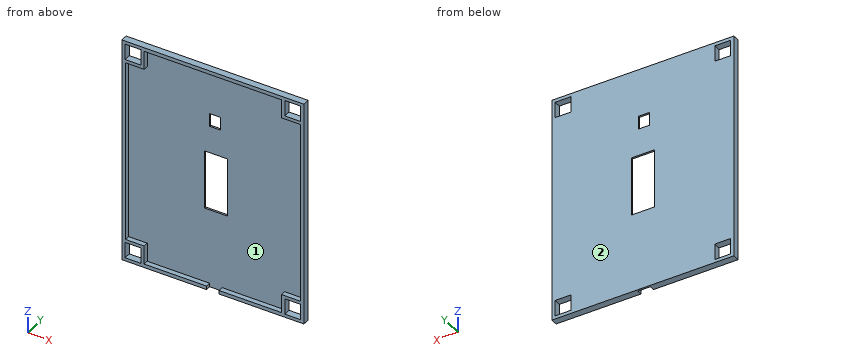
from build123d import *

# Parameters (mm, degrees)
SKETCH1_W           = 80
SKETCH1_H           = 100
BOSS_EXTRUDE1_DEPTH = 3
SKETCH2_W           = 76.8
SKETCH2_H           = 96.8
CUT_EXTRUDE1_DEPTH  = 2.2
CUT_EXTRUDE2_REACH  = 5
SKETCH5_W           = 10
SKETCH5_H           = 26
SKETCH5_W_2         = 4.8
SKETCH5_H_2         = 5.8
SKETCH7_W           = 5.5
SKETCH7_H           = 2.2
CUT_EXTRUDE4_DEPTH  = 3
SKETCH9_W           = 8.2
SKETCH9_H           = 8.2
BOSS_EXTRUDE2_DEPTH = 2.2
SKETCH10_W          = 7
SKETCH10_H          = 7
CUT_EXTRUDE5_DEPTH  = 4


with BuildPart() as part:
    # Sketch1 → Boss-Extrude1 (new body)
    with BuildSketch(Plane(origin=(0, 0, 0), x_dir=(1, 0, 0), z_dir=(0, 1, 0))):
        with Locations((40, 50)):
            Rectangle(SKETCH1_W, SKETCH1_H)
    extrude(amount=BOSS_EXTRUDE1_DEPTH)

    # Sketch2 → Cut-Extrude1 (cut)
    with BuildSketch(Plane.XZ):
        with Locations((40, -50)):
            Rectangle(SKETCH2_W, SKETCH2_H)
    extrude(amount=-CUT_EXTRUDE1_DEPTH, mode=Mode.SUBTRACT)

    # Sketch5 → Cut-Extrude2 (cut, up to next)
    with BuildSketch(Plane(origin=(0, 3, 0), x_dir=(1, 0, 0), z_dir=(0, 1, 0)), mode=Mode.PRIVATE) as cut_extrude2_sk1:
        with Locations((40, 52)):
            Rectangle(SKETCH5_W, SKETCH5_H)
    cut_extrude2_tool1 = extrude(cut_extrude2_sk1.sketch, amount=-CUT_EXTRUDE2_REACH, mode=Mode.PRIVATE) & part.part
    add(cut_extrude2_tool1.solids().sort_by_distance((40, 3, -52))[0], mode=Mode.SUBTRACT)
    # Sketch5 → Cut-Extrude2 (cut, up to next)
    with BuildSketch(Plane(origin=(0, 3, 0), x_dir=(1, 0, 0), z_dir=(0, 1, 0)), mode=Mode.PRIVATE) as cut_extrude2_sk2:
        with Locations((39.6, 24.1)):
            Rectangle(SKETCH5_W_2, SKETCH5_H_2)
    cut_extrude2_tool2 = extrude(cut_extrude2_sk2.sketch, amount=-CUT_EXTRUDE2_REACH, mode=Mode.PRIVATE) & part.part
    add(cut_extrude2_tool2.solids().sort_by_distance((39.6, 3, -24.1))[0], mode=Mode.SUBTRACT)

    # Sketch7 → Cut-Extrude4 (cut)
    with BuildSketch(Plane(origin=(0, 0, -100), x_dir=(-1, 0, 0), z_dir=(0, 0, -1))):
        with Locations((-40, 1.1)):
            Rectangle(SKETCH7_W, SKETCH7_H)
    extrude(amount=-CUT_EXTRUDE4_DEPTH, mode=Mode.SUBTRACT)

    # Sketch9 → Boss-Extrude2 (add)
    with BuildSketch(Plane.XZ.offset(-2.2)):
        with Locations((5.7, -5.7)):
            Rectangle(SKETCH9_W, SKETCH9_H)
        with Locations((74.3, -5.7)):
            Rectangle(SKETCH9_W, SKETCH9_H)
        with Locations((5.7, -94.3)):
            Rectangle(SKETCH9_W, SKETCH9_H)
        with Locations((74.3, -94.3)):
            Rectangle(SKETCH9_W, SKETCH9_H)
    extrude(amount=BOSS_EXTRUDE2_DEPTH)

    # Sketch10 → Cut-Extrude5 (cut, through all)
    with BuildSketch(Plane.XZ):
        with Locations((4.9, -4.9)):
            Rectangle(SKETCH10_W, SKETCH10_H)
        with Locations((4.9, -95.1)):
            Rectangle(SKETCH10_W, SKETCH10_H)
        with Locations((75.1, -95.1)):
            Rectangle(SKETCH10_W, SKETCH10_H)
        with Locations((75.1, -4.9)):
            Rectangle(SKETCH10_W, SKETCH10_H)
    extrude(amount=-CUT_EXTRUDE5_DEPTH, mode=Mode.SUBTRACT)


solid = part.part
Work out the finished part from the listing and answer in its coordinate system (mm). Face numbers are marked on the shaded views. Give positions to 0.01 mm unless a question says otherwise; leave off trailing zeros. Order: outer loops, then holes, each group sorted by start corner. A loop starts at its lowest first (then second) coordinate and runs counter-clockwise, first axis right, second up. Notation, with made-up numbers: (39, 46) -> (45, 46) arc R22 ccw to (45, 72) -> close; hole circle Ø10 at (-18.5, 67.5). An arc over 180 degrees is marked (long way). One line per item, written item: value.
Item 1: Straight lines are drawn through the part: probe 1 along Z at (x, y) = (76.5, 0.7); probe 2 along Z at (x, y) = (61, 2.05); probe 3 along X at (y, z) = (1.1, -73). For each, find the intervals that lie inside material, in ascending order.
Answer sheet:
probe 1: -100 to -98.6, -91.6 to -90.2, -9.8 to -8.4, -1.4 to 0
probe 2: -100 to -98.4, -1.6 to 0
probe 3: 0 to 1.6, 78.4 to 80
Item 2: Flat-ended cylindrical pins translate along their axes: P1, Ø1.5, axis at x = 76, y = 1, coming from the +Z side; P2, Ø1.5, axis at x = 40.5, y = 1, coming from the -Z side; P3, Ø4, axis at x = 15, z = -48.5, coming from the -Y side. Find the tip coordinate at first contact, or state that the pin passes through.
Answer sheet:
P1: z = 0
P2: z = -1.6
P3: y = 2.2
Item 3: Determine the mould class of the marked faces 1 and 2 for opening direction Z: released by +Z, released by -Z, zero draft, split by the parting line, or undercut.
Answer sheet:
face 1: undercut
face 2: zero draft
Item 4: Find section B-B, the plane x = 69. Give the vertices of the cut face in (y, z).
Answer sheet:
outline: (0, -100) -> (3, -100) -> (3, 0) -> (0, 0) -> (0, -1.6) -> (2.2, -1.6) -> (2.2, -98.4) -> (0, -98.4) -> close
Item 5: Find section D-D, the plane y = 1.6. State how many separate pieces and enclosed holes the cut face has, plus the area to 3 significant figures.
Answer sheet:
separate pieces: 1
enclosed holes: 4
area: 630 mm²
Item 6: Find section C-C, the plane z = -85. Give the vertices of the cut face in (x, y).
Answer sheet:
outline: (0, 0) -> (1.6, 0) -> (1.6, 2.2) -> (78.4, 2.2) -> (78.4, 0) -> (80, 0) -> (80, 3) -> (0, 3) -> close
Item 7: Find section A-A, the plane z = -59. Give the vertices of the cut face in (x, y).
Answer sheet:
outline: (0, 0) -> (1.6, 0) -> (1.6, 2.2) -> (35, 2.2) -> (35, 3) -> (0, 3) -> close; (45, 2.2) -> (78.4, 2.2) -> (78.4, 0) -> (80, 0) -> (80, 3) -> (45, 3) -> close
